Input: part model. Units: mm. Frame: model coordinates. A direction names the side the tool comes from. Round coordinates to 2 decimals unless told otherwise and drop trailing zeros. Write each loop counter-clockwise with the first axis right and the second up, starting at its lowest first coordinate (ties: lowest second). Pieces come first, ordered by that corner, then holes. Notation, with made-up numbers: (39.5, -1.75) - (69.5, -1.75) arc R24 cw to (69.5, 21.25) - close; hole circle Ø11 at (-18.5, 28.5). An arc over 180 degrees is marked (long way). Use one line per item in the form item = value.
```python
from build123d import *

# Parameters (mm, degrees)
AUFSATZ_LINEAR_AUSTRAGEN1_DEPTH = 10
AUFSATZ_LINEAR_AUSTRAGEN2_DEPTH = 10
AUFSATZ_LINEAR_AUSTRAGEN3_DEPTH = 10


with BuildPart() as part:
    # Skizze1 → Aufsatz-Linear austragen1 (new body)
    with BuildSketch(Plane.XY):
        Polygon((0, 29.5), (-1.8, 28.5), (-3, -2), (31, -2), (29.8, 28.5), (28, 29.5), (24.7, 28.5), (24.7, 28), (28, 28), (28, 0), (0, 0), (0, 28), (3.3, 28), (3.3, 28.5), align=None)
    extrude(amount=AUFSATZ_LINEAR_AUSTRAGEN1_DEPTH)

    # Skizze1<3> → Aufsatz-Linear austragen2 (add)
    with BuildSketch(Plane.XY):
        Polygon((-2.527868852, 10), (-2.409836066, 13), (-13.5, -2), (-12.105255888, -17.4), (-10.257932824, -18.2), (-8.5, -17), (-10.5, -17), (-10.5, -2), align=None)
        Polygon((30.527868852, 10), (38.5, -2), (38.5, -17), (36.5, -17), (38.257932824, -18.2), (40.105255888, -17.4), (41.5, -2), (30.409836066, 13), align=None)
    extrude(amount=AUFSATZ_LINEAR_AUSTRAGEN2_DEPTH)

    # Skizze1<4> → Aufsatz-Linear austragen3 (add)
    with BuildSketch(Plane.XY):
        Polygon((-3, -2), (-2.921311475, 0), (-9.171311475, 0), (-10.5, -2), align=None)
        Polygon((30.921311475, 0), (31, -2), (38.5, -2), (37.171311475, 0), align=None)
    extrude(amount=AUFSATZ_LINEAR_AUSTRAGEN3_DEPTH)


solid = part.part
```
(1) Cut plane C-C on y = -10. Output: boundary loops of the cut face in (x, z).
Derived:
outline = (-12.78, 0) - (-10.5, 0) - (-10.5, 10) - (-12.78, 10) - close; (38.5, 0) - (40.78, 0) - (40.78, 10) - (38.5, 10) - close
(2) Access query for faces 4 (the face through (30.727, 4.93, 4.93)), 5 (the face through (26.373, 29.007, 4.93)), 6 (the face through (28.9, 29, 4.9)). Directions: +Z, -Z, +X, -X, +Y, -Y. A direction counts if a zero-diameter tool reaches every point of the face in a straight line with its end or side. Return the directions, or none.
Derived:
face_4 = +Z, -Z
face_5 = +Z, -Z, +Y
face_6 = +Z, -Z, +X, +Y
(3) Draft query along X for faces 1 (the face through (-7.88, 5.6, 4.93)), 2 (the face through (1.673, 28.993, 4.93)), 3 (the face through (14, -1, 10)). Return one class per face: released by +X, released by -X, zero draft, split by the parting line, or undercut.
Derived:
face_1 = released by -X
face_2 = undercut
face_3 = zero draft
(4) Cut plane B-B on x = 2.5. Output: boundary loops of the cut face in (y, z), then the cut area to 3 significant figures.
Derived:
outline = (-2, 0) - (0, 0) - (0, 10) - (-2, 10) - close; (28, 0) - (28.74, 0) - (28.74, 10) - (28, 10) - close
area = 27.4 mm^2
(5) Cut plane D-D on y = 4. Output: boundary loops of the cut face in (x, z), then the cut area to 3 significant figures.
Derived:
outline = (-9.06, 0) - (-6.51, 0) - (-6.51, 10) - (-9.06, 10) - close; (-2.76, 0) - (0, 0) - (0, 10) - (-2.76, 10) - close; (28, 0) - (30.76, 0) - (30.76, 10) - (28, 10) - close; (34.51, 0) - (37.06, 0) - (37.06, 10) - (34.51, 10) - close
area = 106 mm^2
(6) Cut plane A-A on z = 5. Count the separate pieces of the cut face and the enclosed holes in it, then the cut area to 3 significant figures.
Derived:
separate_pieces = 1
enclosed_holes = 2
area = 381 mm^2
(7) Material intervals for L1, parallel to X at y = 2, z = 8.5; L2, parallel to X at y = 3.5, z = 9; L3, parallel to Y at x = 16, z = 3, sorted ascending.
Derived:
L1 = -10.54 to -7.84, -2.84 to 0, 28 to 30.84, 35.84 to 38.54
L2 = -9.43 to -6.85, -2.78 to 0, 28 to 30.78, 34.85 to 37.43
L3 = -2 to 0
(8) First-contact query: pin 1 Ø3 at (x, z) = (-6.5, 3) entering from +Y; pin 2 Ø1.6 at (x, z) = (-9, 6.5) entering from +Y; pin 3 Ø1 at (x, z) = (37.5, 5) entering from +Y; pin 4 Ø12 at (x, y) = (27.5, -9) entering from +Z. Flat tips, straight axial feed; report the tip coordinate or a pass-through.
Derived:
pin_1 = 9.5
pin_2 = 5.17
pin_3 = 4.09
pin_4 = through
